Check sheet for the modelled part. Datum: model origin and axes. Units: mm. A direction names the side the tool comes from. Round coordinates to 2 decimals unless told otherwise and drop trailing zeros. Loops run counter-clockwise (first coordinate to the right, second up) from the corner with the lowest first, then second, coordinate; pieces in that order, holes last. Notation, with made-up numbers: (33.5, 57) -> (89.5, 57) arc R19 cw to (89.5, 93) -> close; hole circle Ø5 at (36, 4.5). An arc over 180 degrees is marked (long way). Return JSON: item names as keys, results as strings.
from build123d import *

# Parameters (mm, degrees)
SKETCH1_W             = 19.05
SKETCH1_H             = 23.8125
BOSS_EXTRUDE1_DEPTH   = 4.7625
SKETCH6_R             = 8.5725
CUT_EXTRUDE4_DEPTH    = 5.7625
F_6_CLEARANCE_HOLE1_D = 4.3053
FILLET1_R             = 1.5875


with BuildPart() as part:
    # Sketch1 → Boss-Extrude1 (new body)
    with BuildSketch(Plane.XY):
        Polygon((1.5875, -17.78), (1.5875, -95.5675), (39.1795, -95.5675), (44.1325, -84.455), (44.1325, -17.78), align=None)
        with Locations((22.86, -68.54825)):
            Rectangle(SKETCH1_W, SKETCH1_H, mode=Mode.SUBTRACT)
    extrude(amount=BOSS_EXTRUDE1_DEPTH)

    # Sketch6 → Cut-Extrude4 (cut, through all)
    with BuildSketch(Plane(origin=(156.406140968, -462.385138809, 4.7625), x_dir=(1, 0, 0), z_dir=(0, 0, 1))):
        with Locations((-137.673640968, 421.491138809)):
            Circle(SKETCH6_R)
    extrude(amount=-CUT_EXTRUDE4_DEPTH, mode=Mode.SUBTRACT)

    # #6 Clearance Hole1 (through all)
    with Locations(Plane.XY.offset(4.7625)):
        with Locations((36.1315, -33.274), (29.5275, -88.7095)):
            Hole(F_6_CLEARANCE_HOLE1_D / 2)

    # Fillet1
    fillet1_edges = [part.edges().sort_by_distance(p)[0] for p in [
        (13.335, -80.4545, 2.38125),
        (32.385, -80.4545, 2.38125),
        (32.385, -56.642, 2.38125),
        (13.335, -56.642, 2.38125),
    ]]
    fillet(fillet1_edges, radius=FILLET1_R)


solid = part.part
Q1. Material ranges on line 1 (X direction, y = -59, z = 0.55) (1 decimal); line 2 (Y direction, x = 17, z = 2.95); line 3 (Y direction, x = 16, z = 1.75), recorded low to high.
Results list:
{"line 1": "1.6 to 13.3, 32.4 to 44.1", "line 2": "-95.57 to -80.45, -56.64 to -49.29, -32.5 to -17.78", "line 3": "-95.57 to -80.45, -56.64 to -49.02, -32.77 to -17.78"}
Q2. Section check A-A (y = -63). Record the boundary of the cut face in (x, z) (1 decimal).
Results list:
{"outline": "(1.6, 0) -> (13.3, 0) -> (13.3, 4.8) -> (1.6, 4.8) -> close; (32.4, 0) -> (44.1, 0) -> (44.1, 4.8) -> (32.4, 4.8) -> close"}
Q3. Section check C-C (y = -39.5). Record the boundary of the cut face in (x, z), then the cut area to 3 significant figures.
Results list:
{"outline": "(1.59, 0) -> (10.27, 0) -> (10.27, 4.76) -> (1.59, 4.76) -> close; (27.19, 0) -> (44.13, 0) -> (44.13, 4.76) -> (27.19, 4.76) -> close", "area": "122 mm^2"}
Q4. Draft check along X on faces 3 (the flat face through (23, -56, 0)), 4 (the cylindrical face through (23.341, -33.666, 2.415)), 5 (the flat face through (41.62, -90.09, 2.35)), 6 (the flat face through (1.588, -56, 2)). Enter one of: released by +X, released by -X, zero draft, split by the parting line, or undercut.
Results list:
{"face 3": "zero draft", "face 4": "undercut", "face 5": "released by +X", "face 6": "released by -X"}
Q5. Go/stop test with a flat-tipped pin: pin 1 (1.5 mm diameter, centred on x = 17.5, y = -86, fed in from -Z). Record where the tip stops, or that it passes through.
Results list:
{"pin 1": "z = 0"}
Q6. Tool access check on faces 1 (the flat face through (44.132, -52, 2)), 2 (the cylindrical face through (13.788, -57.119, 2.415)). Record the directions out of +Z, -Z, +X, -X, +Y, -Y that give a thin tool (end or side, any length) a straight path to the whole face; none if there is none.
Results list:
{"face 1": "+Z, -Z, +X, +Y, -Y", "face 2": "+Z, -Z"}
Q7. Section check B-B (z = 3.35). Record the boundary of the cut face in (x, y) (1 decimal), then the cut area to 3 significant figures.
Results list:
{"outline": "(1.6, -95.6) -> (39.2, -95.6) -> (44.1, -84.5) -> (44.1, -17.8) -> (1.6, -17.8) -> close; hole circle Ø17.1 at (18.7, -40.9); hole (13.3, -78.9) arc R1.6 ccw to (14.9, -80.5) -> (30.8, -80.5) arc R1.6 ccw to (32.4, -78.9) -> (32.4, -58.2) arc R1.6 ccw to (30.8, -56.6) -> (14.9, -56.6) arc R1.6 ccw to (13.3, -58.2) -> close; hole circle Ø4.3 at (29.5, -88.7); hole circle Ø4.3 at (36.1, -33.3)", "area": "2,570 mm^2"}
Q8. Section check D-D (x = 41.5). Record the boundary of the cut face in (y, z), then the cut area to 3 significant figures.
Results list:
{"outline": "(-90.36, 0) -> (-17.78, 0) -> (-17.78, 4.76) -> (-90.36, 4.76) -> close", "area": "346 mm^2"}
